Can you work these out from the model? Positions are in its coordinate system, mm. A direction names the side the tool comes from. Give positions to 0.01 mm unless a question says otherwise; leave off trailing zeros. Write each loop counter-clockwise with the first axis right and the second up, starting at its lowest first coordinate (ties: lowest second). Pieces come first, ordered by that corner, then holes. Notation, with made-up numbers: (19.25, 84) - (37.25, 84) arc R13 cw to (37.25, 91) - close; hole circle Ø8 at (5.5, 26.25). An arc over 180 degrees is marked (long way). Use a Markdown table: item, result. Add a question column.
Autodesk Inventor part; units mm, degrees
ref_plane "YZ Plane" through (0, 0, 0) normal (1, 0, 0) x (0, 1, 0)
ref_plane "XZ Plane" through (0, 0, 0) normal (0, 1, 0) x (-1, 0, 0)
ref_plane "XY Plane" through (0, 0, 0) normal (0, 0, 1) x (1, 0, 0)
sketch "Sketch1" plane through (0, 0, 0) normal (0, 0, 1) x (1, 0, 0)
  line L0 (0, 0) -> (50, 0)
  line L1 (50, 0) -> (50, 38)
  line L2 (50, 38) -> (0, 38)
  line L3 (0, 38) -> (0, 0)
  dimension "d0" = 100
  dimension "d1" = 38
revolve "Revolution1" add sketch "Sketch1" angle 360 about axis through (0, 38, 0) along (0, -1, 0)
sketch "Sketch2" plane through (0, 38, 0) normal (0, 1, 0) x (1, 0, 0)
  line L0 (-30, 10) -> (10, 10)
  line L1 (10, 10) -> (10, -10)
  line L2 (10, -10) -> (-30, -10)
  line L3 (-30, -10) -> (-30, 10)
  line L4 (10, -10) -> (17, -10)
  line L5 (17, -10) -> (17, 10)
  line L6 (17, 10) -> (10, 10)
  line L7 (10, 10) -> (10, -10)
  line L8 (-30, -10) -> (-37, -10)
  line L9 (-37, -10) -> (-37, 10)
  line L10 (-37, 10) -> (-30, 10)
  line L11 (-30, 10) -> (-30, -10)
  point P0 (0, 0)
  dimension "d3" = 10
  dimension "d4" = 40
  dimension "d5" = 20
  dimension "d6" = 10
  dimension "d7" = 7
  dimension "d8" = 7
extrude "Extrusion1" cut sketch "Sketch2" against normal blind 38 contours L0 L1 L2 L3
extrude "Extrusion2" cut sketch "Sketch2" against normal blind 10 contours L3 L8 L9 L10 | L6 L5 L4 L1
sketch "Sketch3" plane through (0, 0, 0) normal (0, -1, 0) x (1, 0, 0)
  line L0 (10, 10) -> (10, -10)
  line L1 (10, 6) -> (10, -6)
  line L2 (10, -6) -> (49.6387, -6)
  line L3 (10, 6) -> (49.6387, 6)
  circle A0 centre (0, 0) radius 50
  point P0 (0, 0)
  dimension "d13" = 12
  dimension "d14" = 6
extrude "Extrusion3" cut sketch "Sketch3" against normal blind 10 contours L3 A0 L2 L0 picked at (23.3333, 0)
sketch "Sketch4" plane through (-30, 0, -10) normal (0, -1, 0) x (1, 0, 0)
  line L0 (181, -17) -> (112, -17)
  line L1 (112, -17) -> (112, 37)
  line L2 (112, 37) -> (181, 37)
  line L3 (181, 37) -> (181, -17)
  line L4 (181, -17) -> (112, -17) construction
  line L5 (112, -17) -> (112, 37) construction
  line L6 (112, 37) -> (181, 37) construction
  line L7 (181, 37) -> (181, -17) construction
  line L8 (105, -24) -> (188, -24) construction
  line L9 (188, -24) -> (188, 44) construction
  line L10 (188, 44) -> (105, 44) construction
  line L11 (105, 44) -> (105, -24) construction
  line L12 (105, 44) -> (80, 44) construction
  line L13 (80, 44) -> (80, -24) construction
  line L14 (80, -24) -> (105, -24) construction
  line L15 (105, -24) -> (105, 44)
  arc A0 (79.6387, 4) -> (79.6387, 16) centre (30, 10) ccw
  arc A1 (79.6387, 16) -> (79.6387, 4) centre (30, 10) ccw
  circle A2 centre (30, 41) radius 10
  line L16 (30, 51) -> (53, 51)
  line L17 (58, 46) -> (58, 16)
  line L18 (40, 16) -> (79.6387, 16)
  line L19 (43, 28) -> (43, 16)
  line L20 (30, 10) -> (30, 41) construction
  arc A3 (58, 46) -> (53, 51) centre (53, 46) ccw
  arc A4 (43, 28) -> (40, 31) centre (40, 28) ccw
  circle A5 centre (30, 10) radius 50
  line L21 (30, 60) -> (170, 60)
  line L22 (30, -40) -> (170, -40)
  arc A6 (170, -40) -> (170, 60) centre (170, 10) ccw
  line L23 (40, 31) -> (30, 31)
  point P0 (58, 51)
  dimension "d17" = 69
  dimension "d18" = 54
  dimension "d19" = 7
  dimension "d20" = 25
  dimension "d21" = 34
  dimension "d22" = 20
  dimension "d23" = 15
  dimension "d25" = 28
  dimension "d26" = 35
  dimension "d27" = 5
  dimension "d28" = 3
  dimension "d33" = 100
  dimension "d34" = 50
  dimension "d35" = 140
extrude "Extrusion4" cut sketch "Sketch4" against normal up to surface (10 mm away) contours L18 L19 A4 L23 A2 L16 A3 L17 | A2
sketch "Sketch5" plane through (0, 10, 0) normal (0, -1, 0) x (1, 0, 0)
  circle A0 centre (0, 31) radius 10
  arc A1 (0, 41) -> (0, 21) centre (0, 31) ccw
  point P0 (0, 0)
  dimension "d39" = 20
extrude "Extrusion5" cut sketch "Sketch5" against normal through all
extrude "Extrusion6" add sketch "Sketch4" along normal blind 3 contours L0 L1 L2 L3 | L18 L19 A4 L23 A2 L16 A3 L17 | A1 A0 | A0 A1 L21 A6 L22 | A2
sketch "Sketch6" plane through (0, 38, 0) normal (0, 1, 0) x (1, 0, 0)
  line L0 (-37, -10) -> (-37, 10)
  line L1 (17, -10) -> (-37, -10)
  line L2 (-37, 10) -> (17, 10)
  line L3 (17, 10) -> (17, -10)
  circle A0 centre (0, -31) radius 10
  circle A1 centre (0, -31) radius 10
  line L4 (17, -10) -> (-37, -10)
  line L5 (-37, -10) -> (-37, 10)
  line L6 (-37, 10) -> (17, 10)
  line L7 (17, 10) -> (17, -10)
  circle A2 centre (0, 0) radius 50
  circle A3 centre (0, 0) radius 47
  point P0 (0, 0)
  dimension "d40" = 94
extrude "Extrusion7" add sketch "Sketch6" along normal blind 4 contours A3
equation "\"d34\" = 0.5 * d33"
equation "\"d39\" = d22"
properties part number "Base v0,1"
Q1. I'm going to push flat-ended pins straight in: P1, Ø3, axis at x = 85.5, z = 36, coming from the +Y side; P2, Ø12.5, axis at x = -18.5, y = 30, coming from the +Z side; P3, Ø1.5, axis at x = 11, y = 4.5, coming from the -Z side. Where does each tip first touch, or does it pass through?
Q2. Suppose I cut it at D-D (z = -26). Please give me the cut outline in (x, y), and give its area (3 significant figures).
Q3. On a 3-axis mill with a long thin cutter (end or side, diameter ignored), from which of +Z, -Z, +X, -X, +Y, -Y can I reach the whole of each face in a straight line? I mean faces 4 (the flat face through (30, 5, -6)), 5 (the flat face through (68, -3, 1)), 6 (the flat face through (17, 35, 0)), 7 (the flat face through (5, 5, 21)). Say none if no direction works.
Q4. Suppose I cut it at C-C (x = -22.5). Please give me the cut outline in (y, z), and give its area (3 significant figures).
Q5. If we mould it in two halves opening along X, with no side actions, what happens to faces 1 (the cylindrical face through (189.988, -1.479, 1.099)), 2 (the flat face through (-34, 38, -33)), 3 (the flat face through (-34, 28, 0))? For each: released by +X, released by -X, zero draft, split by the parting line, or undercut.
Q6. Suppose I cut it at A-A (z = 0). Please give me the cut outline in (x, y).
Q7. If I drill on probe 1 along Z at (x, y) = (0, 33.5); probe 2 along X at (y, z) = (31, 31); probe 3 along X at (y, z) = (7, 0), over which ranges is the centre line in solid material (lowest first)? Write a range as [from, to].
Q8. Suppose I cut it at B-B (y = 20). Please give me the cut outline in (x, z).
Derived:
| question | item | result |
|---|---|---|
| 1 | P1 | y = 0 |
| 1 | P2 | z = 48.48 |
| 1 | P3 | z = -48.94 |
| 2 | outline | (-42.71, -3) - (182.71, -3) - (182.71, 0) - (42.71, 0) - (42.71, 38) - (39.15, 38) - (39.15, 42) - (-39.15, 42) - (-39.15, 38) - (-42.71, 38) - close |
| 2 | area | 4,240 mm² |
| 3 | face 4 | +X |
| 3 | face 5 | +Z, -Z, +X, -X, -Y |
| 3 | face 6 | +Y |
| 3 | face 7 | none |
| 4 | outline | (-3, -44.65) - (38, -44.65) - (38, -41.26) - (42, -41.26) - (42, -10) - (0, -10) - (0, 10) - (42, 10) - (42, 41.26) - (38, 41.26) - (38, 44.65) - (-3, 44.65) - close |
| 4 | area | 3,150 mm² |
| 5 | face 1 | released by +X |
| 5 | face 2 | zero draft |
| 5 | face 3 | undercut |
| 6 | outline | (-50, -3) - (190, -3) - (190, 0) - (-30, 0) - (-30, 28) - (-37, 28) - (-37, 42) - (-47, 42) - (-47, 38) - (-50, 38) - close; (10, 10) - (50, 10) - (50, 38) - (47, 38) - (47, 42) - (17, 42) - (17, 28) - (10, 28) - close |
| 7 | probe 1 | [-50, -10], [10, 21], [41, 50] |
| 7 | probe 2 | [-39.23, -10], [10, 39.23] |
| 7 | probe 3 | [-50, -30] |
| 8 | outline | circle Ø100 at (0, 0); hole (-30, -10) - (10, -10) - (10, 10) - (-30, 10) - close; hole circle Ø20 at (0, 31) |
